Build history of the part. All positions in model axes, mm. A direction names the side the tool comes from. Round coordinates to 2 decimals unless told otherwise and drop trailing zeros. Write each loop counter-clockwise with the first axis right and the second up, starting at its lowest first coordinate (ties: lowest second). Pieces come first, ordered by that corner, then holes.
from build123d import *

# Parameters (mm, degrees)
CROQUIS1_W                  = 50.8
CROQUIS1_H                  = 76.2
SALIENTE_EXTRUIR1_DEPTH     = 18
CROQUIS2_W                  = 50.8
CROQUIS2_H                  = 76.2
CROQUIS2_W_2                = 46.12
CROQUIS2_H_2                = 71.52
CROQUIS2_W_3                = 38.8
CROQUIS2_H_3                = 64.2
CORTAR_EXTRUIR1_DEPTH       = 15
CORTAR_EXTRUIR8_DEPTH       = 15
SALIENTE_EXTRUIR3_DEPTH     = 41.5
CORTAR_EXTRUIR9_DEPTH       = 51.5
CORTAR_EXTRUIR10_DEPTH      = 51.5
SALIENTE_EXTRUIR4_DEPTH     = 16
CORTAR_EXTRUIR11_DEPTH      = 16.5
REDONDEO3_R                 = 2
REDONDEO4_R                 = 1
CROQUIS15_W                 = 48.12
CROQUIS15_H                 = 10
CORTAR_EXTRUIR12_DEPTH      = 15
CROQUIS16_W                 = 8
CROQUIS16_H                 = 1.5
CORTAR_EXTRUIR13_DEPTH      = 2
CORTAR_EXTRUIR16_DEPTH      = 49.184748624
CORTAR_EXTRUIR16_DEPTH_BACK = 49.184748624
CROQUIS18_R                 = 10
CROQUIS18_W                 = 2.5
CROQUIS18_H                 = 4.99
CROQUIS18_H_2               = 5.01
CROQUIS19_W                 = 5
CROQUIS19_H                 = 5
CORTAR_EXTRUIR17_DEPTH      = 49.184748624


with BuildPart() as part:
    # Croquis1 → Saliente-Extruir1 (new body)
    with BuildSketch(Plane.XY):
        Rectangle(CROQUIS1_W, CROQUIS1_H)
    extrude(amount=SALIENTE_EXTRUIR1_DEPTH)

    # Croquis2 → Cortar-Extruir1 (cut)
    # profile 1 of 2: a face of its own
    with BuildSketch(Plane.XY.offset(18)):
        Rectangle(CROQUIS2_W, CROQUIS2_H)
        Rectangle(CROQUIS2_W_2, CROQUIS2_H_2, mode=Mode.SUBTRACT)
    # profile 2 of 2: a face of its own
    with BuildSketch(Plane.XY.offset(18)):
        Rectangle(CROQUIS2_W_3, CROQUIS2_H_3)
    extrude(amount=-CORTAR_EXTRUIR1_DEPTH, mode=Mode.SUBTRACT)

    # Croquis6 → Cortar-Extruir8 (cut)
    with BuildSketch(Plane.XY.offset(18)):
        Polygon((-23.06, 35.76), (-8.06, 35.76), (-8.06, 32.1), (-19.4, 32.1), (-19.4, 20.76), (-23.06, 20.76), align=None)
        Polygon((23.06, 35.76), (8.06, 35.76), (8.06, 32.1), (19.4, 32.1), (19.4, 20.76), (23.06, 20.76), align=None)
        Polygon((-23.06, -35.76), (-23.06, -20.76), (-19.4, -20.76), (-19.4, -32.1), (-8.06, -32.1), (-8.06, -35.76), align=None)
        Polygon((23.06, -35.76), (8.06, -35.76), (8.06, -32.1), (19.4, -32.1), (19.4, -20.76), (23.06, -20.76), align=None)
    extrude(amount=-CORTAR_EXTRUIR8_DEPTH, mode=Mode.SUBTRACT)

    # Croquis10 → Saliente-Extruir3 (add)
    with BuildSketch(Plane(origin=(0, -20.76, 0), x_dir=(-1, 0, 0), z_dir=(0, -1, 0))):
        Polygon((23.06, -18), (24.06, -18), (23.06, -3), align=None)
        Polygon((-23.06, -18), (-24.06, -18), (-23.06, -3), align=None)
    extrude(amount=-SALIENTE_EXTRUIR3_DEPTH)

    # Croquis11 → Cortar-Extruir9 (cut)
    with BuildSketch(Plane.XZ.offset(20.76)):
        Polygon((-19.4, 18), (-21.56, 18), (-20.56, 3), (-19.4, 3), align=None)
    extrude(amount=-CORTAR_EXTRUIR9_DEPTH, mode=Mode.SUBTRACT)

    # Croquis12 → Cortar-Extruir10 (cut)
    with BuildSketch(Plane.XZ.offset(20.76)):
        Polygon((19.4, 18), (19.4, 3), (20.56, 3), (21.56, 18), align=None)
    extrude(amount=-CORTAR_EXTRUIR10_DEPTH, mode=Mode.SUBTRACT)

    # Croquis13 → Saliente-Extruir4 (add)
    with BuildSketch(Plane(origin=(8.06, 0, 0), x_dir=(0, 0, -1), z_dir=(1, 0, 0))):
        Polygon((-18, -35.76), (-18, -37.76), (-3, -35.76), align=None)
        Polygon((-18, 35.76), (-18, 37.76), (-3, 35.76), align=None)
    extrude(amount=-SALIENTE_EXTRUIR4_DEPTH)

    # Croquis14 → Cortar-Extruir11 (cut)
    with BuildSketch(Plane(origin=(8.06, 0, 0), x_dir=(0, 0, -1), z_dir=(1, 0, 0))):
        Polygon((-3, -32.1), (-18, -32.1), (-18, -35.26), (-3, -33.26), align=None)
        Polygon((-18, 32.1), (-18, 35.26), (-3, 33.26), (-3, 32.1), align=None)
    extrude(amount=-CORTAR_EXTRUIR11_DEPTH, mode=Mode.SUBTRACT)

    # Redondeo3
    redondeo3_edges = [part.edges().sort_by_distance(p)[0] for p in [
        (-25.4, 38.1, 1.5),
        (25.4, 38.1, 1.5),
        (25.4, -38.1, 1.5),
        (-25.4, -38.1, 1.5),
    ]]
    fillet(redondeo3_edges, radius=REDONDEO3_R)

    # Redondeo4
    redondeo4_edges = [part.edges().sort_by_distance(p)[0] for p in [
        (0, 38.1, 0),
        (-25.4, 0, 0),
        (25.4, 0, 0),
        (0, -38.1, 0),
        (24.814213562, -37.514213562, 0),
        (-24.814213562, -37.514213562, 0),
        (-24.814213562, 37.514213562, 0),
        (24.814213562, 37.514213562, 0),
    ]]
    fillet(redondeo4_edges, radius=REDONDEO4_R)

    # Croquis15 → Cortar-Extruir12 (cut)
    with BuildSketch(Plane.XY.offset(18)):
        with Locations((0, -0.01)):
            Rectangle(CROQUIS15_W, CROQUIS15_H)
    extrude(amount=-CORTAR_EXTRUIR12_DEPTH, mode=Mode.SUBTRACT)

    # Croquis16 → Cortar-Extruir13 (cut)
    with BuildSketch(Plane.XZ.offset(38.1)):
        with Locations((0, 2.25)):
            Rectangle(CROQUIS16_W, CROQUIS16_H)
    extrude(amount=-CORTAR_EXTRUIR13_DEPTH, mode=Mode.SUBTRACT)

    # Croquis18 → Cortar-Extruir16 (cut, two sides: drawn at the far end of the back side and taken through both)
    with BuildSketch(Plane.XY.offset(3).offset(-CORTAR_EXTRUIR16_DEPTH_BACK)):
        Circle(CROQUIS18_R)
        with Locations((21.81, -7.505)):
            Rectangle(CROQUIS18_W, CROQUIS18_H)
        with Locations((21.81, 7.495)):
            Rectangle(CROQUIS18_W, CROQUIS18_H_2)
        with BuildLine():
            Line((20.56, 10), (0, 10))
            ThreePointArc((0, 10), (7.071067812, 7.071067812), (10, 0))
            ThreePointArc((10, 0), (7.071067812, -7.071067812), (0, -10))
            Line((0, -10), (20.56, -10))
            Line((20.56, -10), (20.56, -5.01))
            Line((20.56, -5.01), (23.06, -5.01))
            Line((23.06, -5.01), (23.06, -10))
            Line((23.06, -10), (25.4, -10))
            Line((25.4, -10), (25.4, 10))
            Line((25.4, 10), (23.06, 10))
            Line((23.06, 10), (23.06, 4.99))
            Line((23.06, 4.99), (20.56, 4.99))
            Line((20.56, 4.99), (20.56, 10))
        make_face()
    extrude(amount=CORTAR_EXTRUIR16_DEPTH + CORTAR_EXTRUIR16_DEPTH_BACK, mode=Mode.SUBTRACT)

    # Croquis19 → Cortar-Extruir17 (cut, through all)
    with BuildSketch(Plane.XY.offset(3)):
        with Locations((12.9, 12.5)):
            Rectangle(CROQUIS19_W, CROQUIS19_H)
        with Locations((12.9, -12.5)):
            Rectangle(CROQUIS19_W, CROQUIS19_H)
    extrude(amount=-CORTAR_EXTRUIR17_DEPTH, mode=Mode.SUBTRACT)


solid = part.part
1) Slice it at D-D (x = 9.5). Write the cut outline in (y, z).
Results:
outline: (-38.1, 1) arc R1 ccw to (-37.1, 0) - (-10, 0) - (-10, 3) - (-38.1, 3) - close; (10, 0) - (37.1, 0) arc R1 ccw to (38.1, 1) - (38.1, 3) - (10, 3) - close
2) Slice it at C-C (y = -18.5). Write the cut outline in (x, z), plus the area to 3 significant figures.
Results:
outline: (-25.4, 1) arc R1 ccw to (-24.4, 0) - (24.4, 0) arc R1 ccw to (25.4, 1) - (25.4, 3) - (23.06, 3) - (24.06, 18) - (21.56, 18) - (20.56, 3) - (-20.56, 3) - (-21.56, 18) - (-24.06, 18) - (-23.06, 3) - (-25.4, 3) - close
area: 227 mm2
3) Slice it at B-B (x = -2). Write the cut outline in (y, z), plus the area to 3 significant figures.
Results:
outline: (-38.1, 1) arc R1 ccw to (-37.1, 0) - (-9.8, 0) - (-9.8, 3) - (-33.26, 3) - (-35.26, 18) - (-37.76, 18) - (-35.76, 3) - (-36.1, 3) - (-36.1, 1.5) - (-38.1, 1.5) - close; (9.8, 0) - (37.1, 0) arc R1 ccw to (38.1, 1) - (38.1, 3) - (35.76, 3) - (37.76, 18) - (35.26, 18) - (33.26, 3) - (9.8, 3) - close
area: 241 mm2
4) Wall check: L1, parallel to Y at x = 3.5, z = 2; L2, parallel to Y at x = -23, z = 16.75; L3, parallel to Z at x = -16.5, y = 10. Give the ranges that are in metal, low to high.
Results:
L1: y = -36.1 to -10, 10 to 38.1
L2: y = -20.76 to -5.01, 4.99 to 20.76
L3: z = 0 to 3
5) Slice it at A-A (z = 10.25). Count the separate pieces of the cut face and the enclosed holes in it, plus the area to 3 significant figures.
Results:
separate pieces: 6
enclosed holes: 0
area: 213 mm2
6) Which spindle directions (+Z, -Z, +X, -X, +Y, -Y) get a long thin tool onto all of the face, cutting with end or side? Do faces 1 (the flat face through (21.053, 15.305, 10.395)), 2 (the flat face through (-22, -20.76, 10)), 3 (the flat face through (-8.06, -35, 9)), 4 (the flat face through (-23.567, -12.995, 10.605)), 5 (the flat face through (10.4, 12, 2)). Say none if no direction does.
Results:
face 1: +Z, +Y, -Y
face 2: +Z, +X, -X, -Y
face 3: +Z, -X, +Y, -Y
face 4: -X, +Y, -Y
face 5: +Z, -Z
7) Mould opens along Z. For faces 6 (the flat face through (21.053, -15.455, 10.395)), 7 (the flat face through (21, -10, 7)), 8 (the flat face through (-4, -37, 2)) say: released by +Z, released by -Z, zero draft, split by the parting line, or undercut.
Results:
face 6: released by +Z
face 7: zero draft
face 8: undercut
8) Pin check, flat tips, straight feed: pin 1 Ø1 at (y, z) = (-7, 7) entering from +X; pin 2 Ø5 at (y, z) = (-16.5, 12) entering from -X; pin 3 Ø1 at (y, z) = (-11, 4.5) entering from +X; pin 4 Ø1 at (x, z) = (-10, 4) entering from +Y. Stop position of each tip, or through.
Results:
pin 1: stops at x = -20.79
pin 2: stops at x = -23.83
pin 3: stops at x = 23.19
pin 4: passes through
